from build123d import *

# Parameters (mm, degrees)
SKETCH1_R           = 0.75
SKETCH1_W           = 6.25
SKETCH1_H           = 2.9
BOSS_EXTRUDE1_DEPTH = 3


with BuildPart() as part:
    # Sketch1 → Boss-Extrude1 (new body)
    # profile 1 of 6: a face of its own
    with BuildSketch(Plane.XY):
        with BuildLine():
            ThreePointArc((-50, 40.25), (-47.071067812, 47.321067812), (-40, 50.25))
            Line((-40, 50.25), (25, 50.25))
            ThreePointArc((25, 50.25), (32.071067812, 47.321067812), (35, 40.25))
            Line((35, 40.25), (35, -39.75))
            ThreePointArc((35, -39.75), (32.071067812, -46.821067812), (25, -49.75))
            Line((25, -49.75), (-40, -49.75))
            ThreePointArc((-40, -49.75), (-47.071067812, -46.821067812), (-50, -39.75))
            Line((-50, -39.75), (-50, 40.25))
        make_face()
        Polygon((-3.75, -45.25), (3.75, -45.25), (10, -45.25), (15, -45.25), (15, -42.35), (15, 42.35), (15, 45.25), (10, 45.25), (3.75, 45.25), (-3.75, 45.25), (-10, 45.25), (-15, 45.25), (-15, 42.35), (-15, -42.35), (-15, -45.25), (-10, -45.25), align=None, mode=Mode.SUBTRACT)
    # profile 2 of 6: a face of its own
    with BuildSketch(Plane.XY):
        Polygon((-3.75, -42.35), (3.75, -42.35), (10, -42.35), (15, -42.35), (15, 42.35), (10, 42.35), (3.75, 42.35), (-3.75, 42.35), (-10, 42.35), (-15, 42.35), (-15, -42.35), (-10, -42.35), align=None)
        with Locations((7.5, -22)):
            Circle(SKETCH1_R, mode=Mode.SUBTRACT)
        with Locations((0, -29.5)):
            Circle(SKETCH1_R, mode=Mode.SUBTRACT)
        with Locations((-7.5, -22)):
            Circle(SKETCH1_R, mode=Mode.SUBTRACT)
        with Locations((0, -14.5)):
            Circle(SKETCH1_R, mode=Mode.SUBTRACT)
        with Locations((7.5, 0)):
            Circle(SKETCH1_R, mode=Mode.SUBTRACT)
        with Locations((0, -7.5)):
            Circle(SKETCH1_R, mode=Mode.SUBTRACT)
        with Locations((-7.5, 0)):
            Circle(SKETCH1_R, mode=Mode.SUBTRACT)
        with Locations((0, 7.5)):
            Circle(SKETCH1_R, mode=Mode.SUBTRACT)
        with Locations((-7.5, 22)):
            Circle(SKETCH1_R, mode=Mode.SUBTRACT)
        with Locations((0, 14.5)):
            Circle(SKETCH1_R, mode=Mode.SUBTRACT)
        with Locations((7.5, 22)):
            Circle(SKETCH1_R, mode=Mode.SUBTRACT)
        with Locations((0, 29.5)):
            Circle(SKETCH1_R, mode=Mode.SUBTRACT)
    # profile 3 of 6: a face of its own
    with BuildSketch(Plane.XY):
        with Locations((-6.875, 43.8)):
            Rectangle(SKETCH1_W, SKETCH1_H)
    # profile 4 of 6: a face of its own
    with BuildSketch(Plane.XY):
        with Locations((6.875, 43.8)):
            Rectangle(SKETCH1_W, SKETCH1_H)
    # profile 5 of 6: a face of its own
    with BuildSketch(Plane.XY):
        with Locations((-6.875, -43.8)):
            Rectangle(SKETCH1_W, SKETCH1_H)
    # profile 6 of 6: a face of its own
    with BuildSketch(Plane.XY):
        with Locations((6.875, -43.8)):
            Rectangle(SKETCH1_W, SKETCH1_H)
    extrude(amount=BOSS_EXTRUDE1_DEPTH)


solid = part.part
The model under review builds one solid part; all positions refer to its coordinate system, in mm. A direction names the side the tool comes from. Round coordinates to 2 decimals unless told otherwise and drop trailing zeros. Loops run counter-clockwise (first coordinate to the right, second up) from the corner with the lowest first, then second, coordinate; pieces in that order, holes last. Notation, with made-up numbers: M 5,15.5 L 26,15.5 A25 ccw 26,36.5 Z; hole C 18.5,47.5 d10. An arc over 180 degrees is marked long. Answer as a JSON object with one key per item and string values.
Item 1: For line 1 along Y through (x, z) = (14, 0.3); line 2 along X through (y, z) = (43, 1), list the stretches that pass through material, from the lowest coordinate up.
Check sheet entries:
{"line 1": "-49.75 to -45.25, -42.35 to 42.35, 45.25 to 50.25", "line 2": "-49.61 to -15, -10 to -3.75, 3.75 to 10, 15 to 34.61"}
Item 2: The part is to be moulded in two halves that separate along X. For faces 3 (the face through (-7, 1, 3)), 4 (the face through (10, 44, 1)), 5 (the face through (-50, 0, 1)), say which applies: +X half, -X half, draft (parallel to the pull), parting line (faces both ways), or undercut.
Check sheet entries:
{"face 3": "draft", "face 4": "undercut", "face 5": "-X half"}
Item 3: Tool access review of faces 1 (the face through (-7, 1, 0)), 2 (the face through (-3.75, 44, 1)): name each direction out of +Z, -Z, +X, -X, +Y, -Y from which nothing blocks a thin tool from reaching the whole face with its end or side.
Check sheet entries:
{"face 1": "-Z, +X, -X, +Y, -Y", "face 2": "+Z, -Z"}
Item 4: Clearance check with flat-ended pins moving along their axes: P1, Ø1.2, axis at x = -7.5, y = 22, coming from the -Z side; P2, Ø1.5, axis at y = -43.5, z = 1.5, coming from the -X side; P3, Ø1.5, axis at y = 44, z = 2, coming from the +X side. State where each tip first meets the part, or that it passes through.
Check sheet entries:
{"P1": "through", "P2": "x = -49.54", "P3": "x = 34.54"}
Item 5: We need section A-A, the plane x = 12.5. State the section outline as (y, z) points, and give its area (3 significant figures).
Check sheet entries:
{"outline": "M -49.75,0 L -45.25,0 L -45.25,3 L -49.75,3 Z; M -42.35,0 L 42.35,0 L 42.35,3 L -42.35,3 Z; M 45.25,0 L 50.25,0 L 50.25,3 L 45.25,3 Z", "area": "283 mm2"}
Item 6: We need section B-B, the plane z = 1.5. State how many separate pieces and enclosed holes the cut face has, and give its area (3 significant figures).
Check sheet entries:
{"separate pieces": "1", "enclosed holes": "18", "area": "8,290 mm2"}
